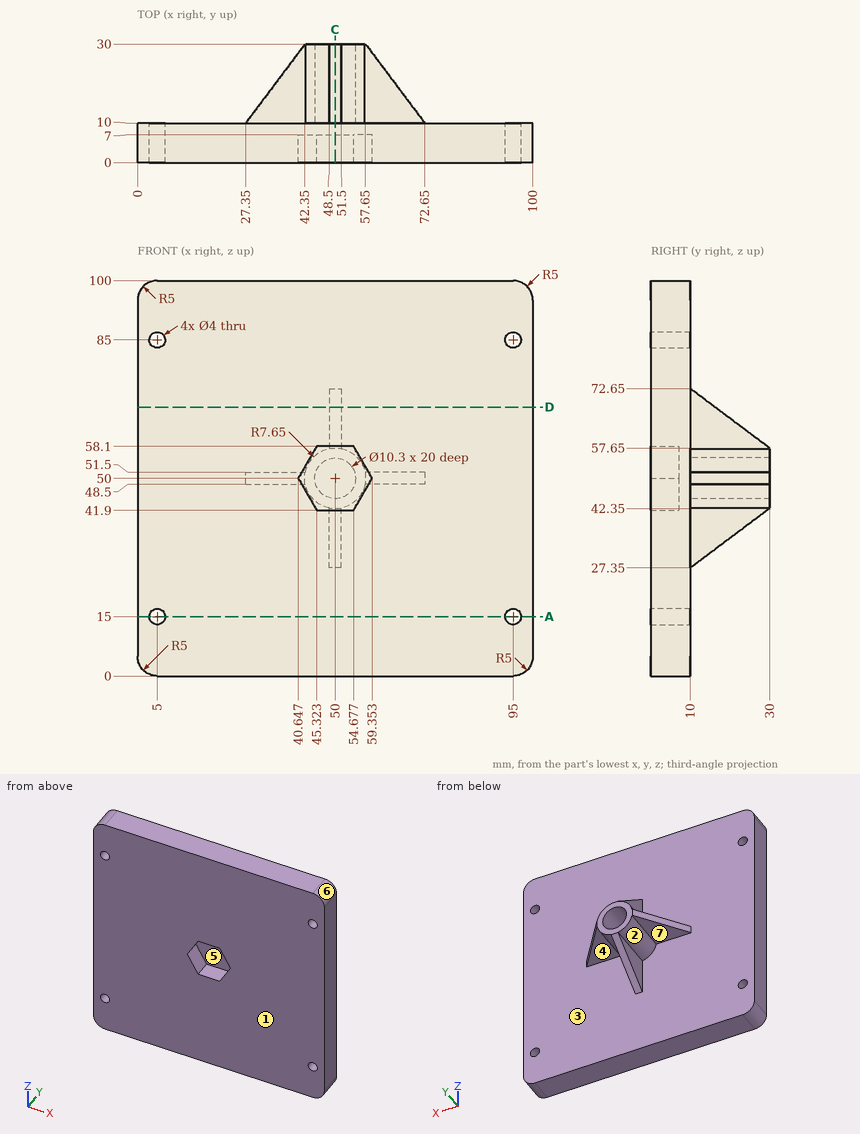
Drawing for the job (mm, zero at the part's lowest x, y, z). A direction names the side the tool comes from. Give positions to 0.01 mm unless a question says otherwise; leave off trailing zeros. Write each loop counter-clockwise with the first axis right and the second up, starting at its lowest first coordinate (ties: lowest second). Pieces come first, ordered by that corner, then holes. Notation, with made-up numbers: M 70.5,30.5 L 86.5,30.5 A15 ccw 86.5,47.5 Z; hole C -25,59 d5. An arc over 180 degrees is marked long. Use CSV: the item, a comma, the result in double quotes.
Item 1: Slice it at D-D on z = 68. Write the cut outline in (x, y), plus the area to 3 significant figures.
Taken from the geometry:
outline,"M 0,0 L 100,0 L 100,10 L 51.5,10 L 51.5,16.2 L 48.5,16.2 L 48.5,10 L 0,10 Z"
area,"1,020 mm²"
Item 2: Pin check, flat tips, straight feed: P1, Ø13.5, axis at x = 50, z = 50, coming from the -Y side; P2, Ø3.5, axis at x = 95, z = 85, coming from the -Y side (3 decimals); P3, Ø4.5, axis at x = 5, z = 15, coming from the +Y side; P4, Ø4.5, axis at y = 20.5, z = 64, coming from the -X side. Stop position of each tip, or through.
Taken from the geometry:
P1,"stops at y = 7"
P2,"passes through"
P3,"stops at y = 10"
P4,"stops at x = 48.5"
Item 3: Drill centre lines: probe 1 along X at (y, z) = (7.5, 15); probe 2 along Y at (x, z) = (64.5, 38); probe 3 along Y at (x, z) = (50.5, 48.5). Where is each one in solid material? Low to high.
Taken from the geometry:
probe 1,"x = 0 to 3, 7 to 93, 97 to 100"
probe 2,"y = 0 to 10"
probe 3,"y = 7 to 10"
Item 4: Slice it at C-C on x = 50. Write the cut outline in (y, z), plus the area to 3 significant figures.
Taken from the geometry:
outline,"M 0,0 L 10,0 L 10,27.35 L 30,42.35 L 30,44.85 L 10,44.85 L 10,55.15 L 30,55.15 L 30,57.65 L 10,72.65 L 10,100 L 0,100 L 0,58.1 L 7,58.1 L 7,41.9 L 0,41.9 Z"
area,"1,290 mm²"
Item 5: Pull direction Z, two halves, no side cores. Call the marked faces 5, 6 and 7: +Z half, -Z half, draft (parallel to the pull), parting line (faces both ways), or undercut.
Taken from the geometry:
face 5,"undercut"
face 6,"+Z half"
face 7,"-Z half"
Item 6: Slice it at A-A on z = 15. Write the cut outline in (x, y), plus the area to 3 significant figures.
Taken from the geometry:
outline,"M 0,0 L 3,0 L 3,10 L 0,10 Z; M 7,0 L 93,0 L 93,10 L 7,10 Z; M 97,0 L 100,0 L 100,10 L 97,10 Z"
area,"920 mm²"
Item 7: Which spindle directions (+Z, -Z, +X, -X, +Y, -Y) get a long thin tool onto all of the face, cutting with end or side? Do the marked faces 1, 2, 3 and 4. Say none if no direction does.
Taken from the geometry:
face 1,"+Z, -Z, +X, -X, -Y"
face 2,"-Z, -X, +Y"
face 3,"+Y"
face 4,"-Z, +X, +Y"
